```python
from build123d import *

# Parameters (mm, degrees)
EXTRUDE_1_DEPTH          = 30
EXTRUDE_1_DEPTH_BACK     = 20
SKETCH_1_W               = 182
SKETCH_1_H               = 6
SKETCH_2_W               = 15.454545454
SKETCH_2_H               = 6
EXTRUDE_2_DEPTH          = 286.2
EXTRUDE_3_DEPTH          = 5
PATTERN_START            = 137.957019682
PATTERN_LINEAR_1_DEPTH   = 6
PATTERN_START_2          = 132.957019682
PATTERN_LINEAR_1_2_DEPTH = 5
SKETCH_6_R               = 2.25
CUT_EXTRUDE_1_DEPTH      = 48835.841869249


# Read off the part's stored shape, not the designer's step: Линейный массив1
with BuildPart() as part:
    # Эскиз1 → Бобышка-Вытянуть1 (new, two sides: drawn at the far end of the back side and taken through both)
    with BuildSketch(Plane(origin=(-714.669316418, 0, -48802.97861783), x_dir=(0.9998927943248835, 0, -0.01464239929711995), z_dir=(0.01464239929711995, 0, 0.9998927943248835)).offset(-EXTRUDE_1_DEPTH_BACK)):
        with Locations((-531.386445276, 140.957019682)):
            Rectangle(SKETCH_1_W, SKETCH_1_H)
    extrude(amount=EXTRUDE_1_DEPTH + EXTRUDE_1_DEPTH_BACK)

    # Эскиз2 → Бобышка-Вытянуть2 (add)
    with BuildSketch(Plane(origin=(-714.23004444, 0, -48772.981834), x_dir=(0.9998927943248835, 0, -0.01464239929711995), z_dir=(0.01464239929711995, 0, 0.9998927943248835))):
        with Locations((-469.568263457, 140.957019682)):
            Rectangle(SKETCH_2_W, SKETCH_2_H)
    extrude(amount=EXTRUDE_2_DEPTH)

    # Эскиз5 → Бобышка-Вытянуть3 (add)
    with BuildSketch(Plane.XZ.offset(-137.957019682)):
        Polygon((-1187.283757155, -48479.82376444), (-1187.371611551, -48485.823121206), (-1171.918722912, -48486.049412832), (-1171.830868516, -48480.050056066), align=None)
    extrude(amount=EXTRUDE_3_DEPTH)

    # Линейный массив1 outline → Линейный массив1 (add)
    with BuildSketch(Plane(origin=(0, 0, 0), x_dir=(1, 0, 0), z_dir=(0, 1, 0)).offset(PATTERN_START)):
        Polygon((-1310.906866272, 48478.013431436), (-1295.453977632, 48478.239723062), (-1299.644632311, 48764.409040798), (-1315.097520951, 48764.182749172), align=None)
        Polygon((-1206.927300474, 48765.766790551), (-1222.380189113, 48765.540498925), (-1218.189534435, 48479.371181189), (-1202.736645795, 48479.597472815), align=None)
        Polygon((-1237.833077753, 48765.3142073), (-1253.285966393, 48765.087915674), (-1249.095311714, 48478.918597939), (-1233.642423074, 48479.144889564), align=None)
        Polygon((-1268.738855032, 48764.861624049), (-1284.191743672, 48764.635332423), (-1280.001088993, 48478.466014687), (-1264.548200353, 48478.692306313), align=None)
    extrude(amount=PATTERN_LINEAR_1_DEPTH)

    # Pattern Linear 1 2 outline → Pattern Linear 1 2 (add)
    with BuildSketch(Plane(origin=(0, 0, 0), x_dir=(1, 0, 0), z_dir=(0, 1, 0)).offset(PATTERN_START_2)):
        Polygon((-1310.994720668, 48484.012788202), (-1310.906866272, 48478.013431436), (-1295.453977632, 48478.239723062), (-1295.541832028, 48484.239079828), align=None)
        Polygon((-1264.636054749, 48484.691663079), (-1280.088943389, 48484.465371453), (-1280.001088993, 48478.466014688), (-1264.548200353, 48478.692306313), align=None)
        Polygon((-1233.73027747, 48485.14424633), (-1249.18316611, 48484.917954704), (-1249.095311714, 48478.918597939), (-1233.642423074, 48479.144889564), align=None)
        Polygon((-1202.824500191, 48485.596829581), (-1218.27738883, 48485.370537955), (-1218.189534435, 48479.371181189), (-1202.736645795, 48479.597472815), align=None)
    extrude(amount=PATTERN_LINEAR_1_2_DEPTH)

    # Эскиз6 → Вырез-Вытянуть1 (cut, through all)
    with BuildSketch(Plane.XZ.offset(-137.957019682)):
        with Locations((-1262.204177172, -48774.958389842)):
            Circle(SKETCH_6_R)
        with Locations((-1229.207714959, -48775.441589019)):
            Circle(SKETCH_6_R)
    extrude(amount=-CUT_EXTRUDE_1_DEPTH, mode=Mode.SUBTRACT)


solid = part.part
```
Check sheet for the modelled part. Datum: model origin and axes. Units: mm. A direction names the side the tool comes from. Coordinates: 2 decimals unless noted, no trailing zeros. Loops run counter-clockwise (first coordinate to the right, second up) from the corner with the lowest first, then second, coordinate; pieces in that order, holes last. Notation, with made-up numbers: M 14.5,7.5 L 18.5,7.5 A24 ccw 18.5,46.5 Z; hole C -18,55.25 d8. An arc over 180 degrees is marked long. Answer as a JSON object with one key per item and string values.
1. Sectioned sample at A-A on y = 136. Record the cut outline in (x, z).
Outcome:
{"outline": "M -1310.99,-48484.01 L -1295.54,-48484.24 L -1295.45,-48478.24 L -1310.91,-48478.01 Z; M -1280.09,-48484.47 L -1264.64,-48484.69 L -1264.55,-48478.69 L -1280,-48478.47 Z; M -1249.18,-48484.92 L -1233.73,-48485.14 L -1233.64,-48479.14 L -1249.1,-48478.92 Z; M -1218.28,-48485.37 L -1202.82,-48485.6 L -1202.74,-48479.6 L -1218.19,-48479.37 Z; M -1187.37,-48485.82 L -1171.92,-48486.05 L -1171.83,-48480.05 L -1187.28,-48479.82 Z"}
2. Sectioned sample at C-C on x = -1320. Record the cut outline in (y, z).
Outcome:
{"outline": "M 137.96,-48814.12 L 143.96,-48814.12 L 143.96,-48764.11 L 137.96,-48764.11 Z"}
3. Sectioned sample at B-B on z = -48500.5. Record the cut outline in (x, y).
Outcome:
{"outline": "M -1311.24,137.96 L -1295.78,137.96 L -1295.78,143.96 L -1311.24,143.96 Z; M -1280.32,137.96 L -1264.87,137.96 L -1264.87,143.96 L -1280.32,143.96 Z; M -1249.41,137.96 L -1233.96,137.96 L -1233.96,143.96 L -1249.41,143.96 Z; M -1218.5,137.96 L -1203.04,137.96 L -1203.04,143.96 L -1218.5,143.96 Z; M -1187.59,137.96 L -1172.13,137.96 L -1172.13,143.96 L -1187.59,143.96 Z"}
4. Depth check by flat-ended pin: P1, Ø6, axis at y = 137, z = -48729.5, coming from the +X side; P2, Ø4, axis at x = -1181.5, z = -48649, coming from the -Y side; P3, Ø5, axis at y = 139.5, z = -48580.5, coming from the +X side; P4, Ø5, axis at x = -1262.2, z = -48774.96, coming from the +Y side. Enter the tip coordinate at first touch or a pass-through.
Outcome:
{"P1": "x = -1175.44", "P2": "y = 137.96", "P3": "x = -1173.27", "P4": "y = 143.96"}
5. Scan lines: L1, parallel to X at y = 139, z = -48559; L2, parallel to X at y = 143.5, z = -48662.5; L3, parallel to Z at x = -1275, y = 135.25. Record each from-to range of solid material in increasing order. Write a range as from..to.
Outcome:
{"L1": "-1312.09..-1296.64, -1281.18..-1265.72, -1250.27..-1234.81, -1219.36..-1203.9, -1188.44..-1172.99", "L2": "-1313.61..-1298.15, -1282.7..-1267.24, -1251.78..-1236.33, -1220.87..-1205.42, -1189.96..-1174.5", "L3": "-48484.54..-48478.54"}
6. Access from +Z, -Z, +X, -X, +Y, -Y to the whole of each face (thin tool, end or side, straight path). Record for faces 1 (the flat face through (-1303, 132.957, -48481)), 2 (the flat face through (-1246, 137.957, -48689)).
Outcome:
{"face 1": "+Z, -Z, +X, -X, -Y", "face 2": "-Z, +X, -X, -Y"}
